Geometry: final body of the model. Coordinates: model frame, mm. A direction names the side the tool comes from. Give positions to 0.01 mm unless a question says otherwise; leave off trailing zeros. Write each loop counter-clockwise with the first axis right and the second up, starting at its lowest first coordinate (ties: lowest second). Pieces come first, ordered by that corner, then holes. Notation, with made-up numbers: M 56.25,12 L 73.25,12 A11 cw 73.25,20 Z; hole C 18,-2 d3. An arc over 180 degrees is marked long. Use a Markdown table: item, result. Add a question column.
1) Section B-B on x = 0. Return the cut outline in (y, z).
2) Set-up query: faces 1 (the flat face through (-6.35, -26, 14)), 2 (the flat face through (-40, 0, 15)), 3 (the flat face through (25, 0, 9.804)). Return all of +Z, -Z, +X, -X, +Y, -Y with unobstructed straight access to the full face (end or side cutting, diameter ignored); none if empty.
3) Pin query (flat end, axial travel): pin 1 (2.5 mm diameter, centred on x = 0.5, y = -27.5, fed in from +Z); pin 2 (0.8 mm diameter, centred on y = -2, z = 13.5, fed in from +X); pin 3 (4 mm diameter, centred on x = -4.5, y = 19, fed in from +Z). Return the tip coordinate at first contact, or that it passes through.
4) Line query: line 1 (X direction, y = 0, z = 5.5); line 2 (Y direction, x = 0, z = 4.75); line 3 (X direction, y = -23.5, z = 14). Output: solid intervals per line, ascending.
5) Section D-D on y = 12.5. Return the cut outline in (x, z).
6) Section A-A on y = 20. Return the cut outline in (x, z), then the cut area to 3 significant figures.
7) Section C-C on z = 11. Return the cut outline in (x, y), then the cut area to 3 significant figures.
8) Draft query along X for faces 4 (the flat face through (45, 0, 2)), 5 (the flat face through (18.5, 22.2, 12.4)), 6 (the cylindrical face through (49.93, -0.651, 12.457)). Return one class per face: +X half, -X half, draft (parallel to the pull), parting line (faces both ways), or undercut.
```python
from build123d import *

# Parameters (mm, degrees)
F0_W     = 90
F0_H     = 60
F0_R     = 22.5
F1_DEPTH = 15
F2_W     = 10
F2_H     = 60
F3_DEPTH = 2.54
F5_DEPTH = 60.001
F6_R     = 5
F7_DEPTH = 10


with BuildPart() as f1:
    # F0 (on Top) → F1 (new body)
    with BuildSketch(Plane.XY):
        Rectangle(F0_W, F0_H)
        Circle(F0_R, mode=Mode.SUBTRACT)
    extrude(amount=F1_DEPTH)

    # F2 (on face) → F3 (cut)
    with BuildSketch(Plane.XY.offset(15)):
        with Locations((-30, 0)):
            Rectangle(F2_W, F2_H)
        with BuildLine():
            Line((6.35, 30), (-6.35, 30))
            Line((-6.35, 30), (-6.35, 21.585354))
            ThreePointArc((-6.35, 21.585354), (0, 22.5), (6.35, 21.585354))
            Line((6.35, 21.585354), (6.35, 30))
        make_face()
        with BuildLine():
            Line((-6.35, -21.585354), (-6.35, -30))
            Line((-6.35, -30), (6.35, -30))
            Line((6.35, -30), (6.35, -21.585354))
            ThreePointArc((6.35, -21.585354), (0, -22.5), (-6.35, -21.585354))
        make_face()
    extrude(amount=-F3_DEPTH, mode=Mode.SUBTRACT)

    # F4 (on face) → F5 (cut, through all)
    with BuildSketch(Plane.XZ.offset(30)):
        Polygon((30, 15), (20, 15), (17, 9.803848), (33, 9.803848), align=None)
    extrude(amount=-F5_DEPTH, mode=Mode.SUBTRACT)

    # F6 (on face) → F7 (join)
    with BuildSketch(Plane.YZ.offset(45)):
        with Locations((0, 7.5)):
            Circle(F6_R)
    extrude(amount=F7_DEPTH)


solid = f1.part
```
Found:
| question | item | result |
|---|---|---|
| 1 | outline | M -30,0 L -22.5,0 L -22.5,12.46 L -30,12.46 Z; M 22.5,0 L 30,0 L 30,12.46 L 22.5,12.46 Z |
| 2 | face 1 | +Z, +Y, -Y |
| 2 | face 2 | +Z, +X, -X, +Y, -Y |
| 2 | face 3 | +Y, -Y |
| 3 | pin 1 | z = 12.46 |
| 3 | pin 2 | x = 45 |
| 3 | pin 3 | through |
| 4 | line 1 | -45 to -22.5, 22.5 to 55 |
| 4 | line 2 | -30 to -22.5, 22.5 to 30 |
| 4 | line 3 | -45 to -35, -25 to -6.35, 6.35 to 19.42, 30.58 to 45 |
| 5 | outline | M -45,0 L -18.71,0 L -18.71,15 L -25,15 L -25,12.46 L -35,12.46 L -35,15 L -45,15 Z; M 18.71,0 L 45,0 L 45,15 L 30,15 L 33,9.8 L 18.71,9.8 Z; M 18.71,12.76 L 20,15 L 18.71,15 Z |
| 6 | outline | M -45,0 L -10.31,0 L -10.31,15 L -25,15 L -25,12.46 L -35,12.46 L -35,15 L -45,15 Z; M 10.31,0 L 45,0 L 45,15 L 30,15 L 33,9.8 L 17,9.8 L 20,15 L 10.31,15 Z |
| 6 | area | 948 mm² |
| 7 | outline | M -45,-30 L 17.69,-30 L 17.69,-13.9 A22.5 cw long 17.69,13.9 L 17.69,30 L -45,30 Z; M 32.31,-30 L 45,-30 L 45,-3.57 L 55,-3.57 L 55,3.57 L 45,3.57 L 45,30 L 32.31,30 Z |
| 7 | area | 3,100 mm² |
| 8 | face 4 | +X half |
| 8 | face 5 | undercut |
| 8 | face 6 | draft |
